Answer from the drawing. Dimensions are ordinates in mm from the lowest x, y and z of the part. Give positions to 0.01 mm unless a question says otherwise; leave off trailing zeros. Loops run counter-clockwise (first coordinate to the right, second up) from the corner with the lowest first, then second, coordinate; pieces in that order, holes last.
Item 1: Each of these flat-tipped pins is pushed along its axis until it touches: pin 1 Ø1.2 at (x, y) = (1, 1.5) entering from +Z; pin 2 Ø6.5 at (x, y) = (5.79, 32.96) entering from -Z. Where does it stop, or does it pass through?
Item 2: Section D-D, the plane y = 41.5 is taken. Give the vertices of the cut face in (x, z).
Item 3: Section C-C, the plane z = 6.5 is taken. Give the number of separate pieces and of enclosed holes in the cut face, and give its area (3 significant figures).
Item 4: The mould has two halves that part along Y. Classify the marked faces 1, 2, 3 and 4: pulls with the +Y half, pulls with the -Y half, needs draft (parallel to the pull), parting line crosses it, or undercut.
Item 5: Consider line 1 along Y through (x, z) = (4.75, 2.75) (1 decimal); line 2 along Y through (x, z) = (5.25, 2.75); line 3 along X through (y, z) = (6.5, 9.25). Determine where each line is inside the solid, lowest interval first.
Item 6: Section A-A, the plane x = 7.5 is taken. Give the vertices of the cut face in (y, z).
Item 7: Section B-B, the plane y = 31.5 is taken. Give the vertices of the cut face in (x, z).
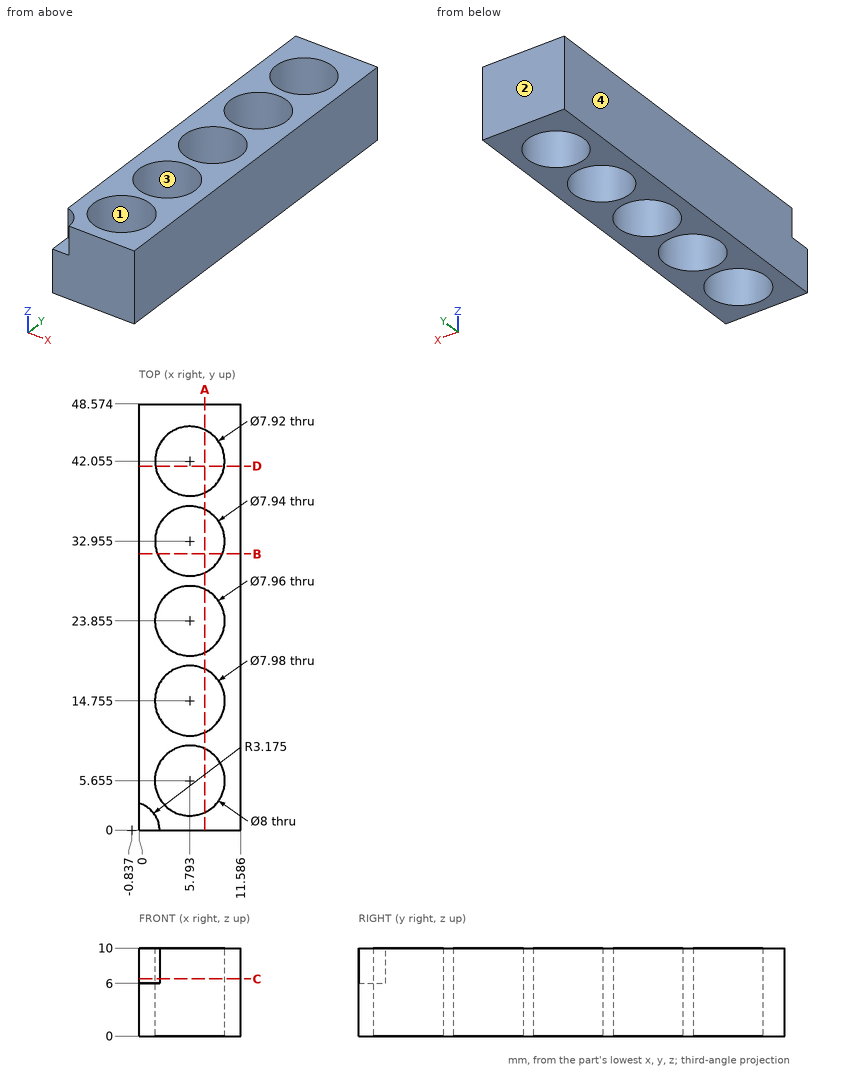
Worked answers:
1. pin 1: stops at z = 6
1. pin 2: passes through
2. outline: (0, 0) - (1.87, 0) - (1.87, 10) - (0, 10) - close; (9.71, 0) - (11.59, 0) - (11.59, 10) - (9.71, 10) - close
3. separate pieces: 1
3. enclosed holes: 5
3. area: 309 mm2
4. face 1: undercut
4. face 2: pulls with the +Y half
4. face 3: undercut
4. face 4: needs draft
5. line 1: y = 0 to 1.8, 9.5 to 10.9, 18.6 to 20, 27.7 to 29.1, 36.8 to 38.2, 45.9 to 48.6
5. line 2: y = 0 to 1.69, 9.62 to 10.8, 18.71 to 19.91, 27.8 to 29.02, 36.89 to 38.13, 45.98 to 48.57
5. line 3: x = 0 to 1.88, 9.7 to 11.59
6. outline: (0, 0) - (2.04, 0) - (2.04, 10) - (0, 10) - close; (9.27, 0) - (11.15, 0) - (11.15, 10) - (9.27, 10) - close; (18.36, 0) - (20.26, 0) - (20.26, 10) - (18.36, 10) - close; (27.45, 0) - (29.37, 0) - (29.37, 10) - (27.45, 10) - close; (36.54, 0) - (38.48, 0) - (38.48, 10) - (36.54, 10) - close; (45.63, 0) - (48.57, 0) - (48.57, 10) - (45.63, 10) - close
7. outline: (0, 0) - (2.1, 0) - (2.1, 10) - (0, 10) - close; (9.49, 0) - (11.59, 0) - (11.59, 10) - (9.49, 10) - close
